Model file for the job. Use its own axes, mm. Round coordinates to 2 decimals unless told otherwise and drop trailing zeros. Order: outer loops, then holes, each group sorted by start corner. A loop starts at its lowest first (then second) coordinate and runs counter-clockwise, first axis right, second up. Notation, with made-up numbers: (85, 56) - (129, 56) arc R14 cw to (129, 79) - close; hole circle Ø11 at (-13.5, -7.75). An arc over 180 degrees is marked (long way). Use one line per item in the form item = value.
from build123d import *

# Parameters (mm, degrees)
REVOLVE_1_ANGLE      = 180
SHELL_1_T            = 0.5
SKETCH_2_OUTSIDE_W   = 328.82
SKETCH_2_OUTSIDE_H   = 328.82
SKETCH_2_OUTSIDE_R   = 75
SKETCH_2_OUTSIDE_R_2 = 57.5
CUT_EXTRUDE_1_DEPTH  = 323


with BuildPart() as part:
    # 草图1 → 旋转1 (revolve)
    with BuildSketch(Plane.XY):
        with BuildLine():
            Line((0, -125.2), (0, 125.2))
            ThreePointArc((0, 125.2), (-125.2, 0), (0, -125.2))
        make_face()
    revolve(axis=Axis((0, 175.755690027, 0), (0, -1, 0)), revolution_arc=REVOLVE_1_ANGLE)

    # 抽壳1
    shell_1_openings = [part.faces().sort_by_distance(p)[0] for p in [
        (0, 0, 0),
    ]]
    offset(amount=SHELL_1_T, openings=shell_1_openings)

    # 草图2 outside → 切除-拉伸1 (cut)
    with BuildSketch(Plane(origin=(0, 0, 0), x_dir=(1, 0, 0), z_dir=(0, 0, -1))):
        Rectangle(SKETCH_2_OUTSIDE_W, SKETCH_2_OUTSIDE_H)
        with Locations(Location((0, 0, 0), (0, 0, 90))):
            Circle(SKETCH_2_OUTSIDE_R, mode=Mode.SUBTRACT)
        with Locations(Location((0, 0, 0), (0, 0, 90))):
            Circle(SKETCH_2_OUTSIDE_R_2)
    extrude(amount=CUT_EXTRUDE_1_DEPTH, mode=Mode.SUBTRACT)


solid = part.part
(1) Slice it at A-A on x = 0. Give the cut face in (y, z).
Report:
outline = (-75, -100.87) arc R125.7 ccw to (-57.5, -111.78) - (-57.5, -111.22) arc R125.2 cw to (-75, -100.25) - close; (57.5, -111.78) arc R125.7 ccw to (75, -100.87) - (75, -100.25) arc R125.2 cw to (57.5, -111.22) - close
(2) Probe probe 1 along Y at (x, z) = (-10.5, -106.5); probe 2 along X at (y, z) = (-30, -101); probe 3 along X at (y, z) = (21, -104.25). List the from-to ranges inside material, lowest first. Write a range as [from, to].
Report:
probe_1 = [-65.94, -64.98], [64.98, 65.94]
probe_2 = [-68.55, -67.63], [67.63, 68.55]
probe_3 = [-67.02, -66.08], [66.08, 67.02]
(3) Slice it at C-C on z = -105.25. Give the cut face in (x, y), then the cut area to 3 significant figures.
Report:
outline = circle Ø137.45 at (0, 0); hole circle Ø135.61 at (0, 0)
area = 394 mm2
(4) Pin check, flat tips, straight feed: pin 1 (4 mm diameter, centred on y = -32.5, z = -104.5, fed in from +X); pin 2 (5 mm diameter, centred on y = 46, z = -109, fed in from +X); pin 3 (2 mm diameter, centred on x = 33.5, z = -103.5, fed in from +Y). Stop position of each tip, or through.
Report:
pin_1 = 65.25
pin_2 = 48.88
pin_3 = 64.67
(5) Pull direction Y, two halves, no side cores. Call faces 1 (the face through (56.133, 12.465, -111.492)), 2 (the face through (45.636, 59.517, -100.557)): released by +Y, released by -Y, zero draft, split by the parting line, or undercut.
Report:
face_1 = undercut
face_2 = split by the parting line
